Read the model definition and answer for the solid it produces. Units are mm, in the model's axes. A direction names the side the tool comes from. Give positions to 0.01 mm unless a question says otherwise; leave off trailing zeros. Write each loop counter-clockwise with the first axis right and the second up, starting at its lowest first coordinate (ties: lowest second). Pieces come first, ordered by that corner, then holes.
```python
from build123d import *

# Parameters (mm, degrees)
SKETCH_W     = 2
SKETCH_H     = 15
PAD_DEPTH    = 15
PAD001_DEPTH = 2


with BuildPart() as part:
    # Sketch → Pad (new body)
    with BuildSketch(Plane.XY):
        with Locations((1, 7.5)):
            Rectangle(SKETCH_W, SKETCH_H)
    extrude(amount=PAD_DEPTH)

    # Sketch001 → Pad001 (join)
    with BuildSketch(Plane.XY.offset(15)):
        with BuildLine():
            Line((0, 18.76349), (2.029385, 18.76349))
            ThreePointArc((6.029385, 14.76349), (4.857812, 17.591917), (2.029385, 18.76349))
            Line((6.029385, 14.76349), (6.029385, 0.208627))
            ThreePointArc((2.029385, -3.791373), (4.857812, -2.6198), (6.029385, 0.208627))
            Line((2.029385, -3.791373), (0, -3.791373))
            ThreePointArc((-4, 0.208627), (-2.828427, -2.6198), (0, -3.791373))
            Line((-4, 0.208627), (-4, 14.76349))
            ThreePointArc((0, 18.76349), (-2.828427, 17.591917), (-4, 14.76349))
        make_face()
    extrude(amount=PAD001_DEPTH)


solid = part.part
```
Item 1: Find the intervals of material crossed by line 1 along Z through (x, y) = (2.75, 5.5); line 2 along X through (y, z) = (14.75, 9.25); line 3 along Y through (x, z) = (1.25, 10.75), in increasing order.
Result set:
line 1: z = 15 to 17
line 2: x = 0 to 2
line 3: y = 0 to 15
Item 2: Section B-B (z = 16) is taken. Write down the section's boundary in (x, y), and give its area (3 significant figures).
Result set:
outline: (-4, 0.21) arc R4 ccw to (0, -3.79) - (2.03, -3.79) arc R4 ccw to (6.03, 0.21) - (6.03, 14.76) arc R4 ccw to (2.03, 18.76) - (0, 18.76) arc R4 ccw to (-4, 14.76) - close
area: 212 mm2
Item 3: Section D-D (z = 11) is taken. Write down the section's boundary in (x, y).
Result set:
outline: (0, 0) - (2, 0) - (2, 15) - (0, 15) - close
Item 4: Section A-A (x = 0.75) is taken. Write down the section's boundary in (y, z).
Result set:
outline: (-3.79, 15) - (0, 15) - (0, 0) - (15, 0) - (15, 15) - (18.76, 15) - (18.76, 17) - (-3.79, 17) - close
Item 5: Each of these flat-tipped pins is pushed along its axis until it touches: pin 1 Ø0.6 at (x, z) = (1, 5) entering from +Y; pin 2 Ø4.5 at (y, z) = (5.5, 4) entering from +X; pin 3 Ø5 at (x, y) = (2.5, 9) entering from -Z; pin 4 Ø1.6 at (x, z) = (1.5, 7) entering from -Y. Where does it stop, or does it pass through?
Result set:
pin 1: stops at y = 15
pin 2: stops at x = 2
pin 3: stops at z = 0
pin 4: stops at y = 0
Item 6: Section C-C (y = 16) is taken. Write down the section's boundary in (x, z).
Result set:
outline: (-3.8, 15) - (5.83, 15) - (5.83, 17) - (-3.8, 17) - close
Item 7: Which of the six approach directions +Z, -Z, +X, -X, +Y, -Y give full straight-line access (tool end or side, diameter ignored) to faces 1 (the flat face through (2, 7, 7)), 2 (the flat face through (1, 15, 7)), 3 (the flat face through (1, 0, 7))?
Result set:
face 1: -Z, +X, +Y, -Y
face 2: -Z, +X, -X, +Y
face 3: -Z, +X, -X, -Y
